Design review of the part built by this model. Coordinates are the model's own, in mm. Give positions to 0.01 mm unless a question says otherwise; leave off trailing zeros. Loops run counter-clockwise (first coordinate to the right, second up) from the corner with the lowest first, then second, coordinate; pieces in that order, holes last. Notation, with made-up numbers: (2.5, 32.25) -> (12.5, 32.25) arc R17 ccw to (12.5, 40.25) -> close; hole circle Ø3 at (32.5, 49). An arc over 180 degrees is marked (long way). Use a Markdown table: item, result. Add a question column.
1. Add section D-D (z = 2). State the section outline as (x, y) points.
2. For pin 1 Ø5 at (y, z) = (10, 6.5) entering from +X; pin 2 Ø4 at (y, z) = (6.5, -2) entering from +X, all flat-tipped, find the tip position at first contact; note any pin that passes through.
3. To check wall thickness, follow line 1 (Y direction, x = 55, z = -1.25); line 2 (Y direction, x = 55.5, z = 3); line 3 (X direction, y = 14.5, z = -4.5). State the ranges of each line that lie inside material, in increasing order.
4. Add section C-C (z = -1). State the section outline as (x, y) points.
5. Add section A-A (x = 55.3). State the section outline as (y, z) points, and give its area (3 significant figures).
6. Add section B-B (y = 11). State the section outline as (x, z) points, and give its area (3 significant figures).
```python
from build123d import *

# Parameters (mm, degrees)
BOSS_EXTRUDE1_DEPTH = 15
CUT_EXTRUDE1_DEPTH  = 40


with BuildPart() as part:
    # Sketch2 → Boss-Extrude1 (new body)
    with BuildSketch(Plane(origin=(0, 0, 0), x_dir=(1, 0, 0), z_dir=(0, 1, 0))):
        with BuildLine():
            Line((54.845806585, -8.617162068), (54.845806585, -10))
            ThreePointArc((54.845806585, -10), (55.523491502, -5.020397537), (55.75, 0))
            Line((55.75, 0), (55.518627344, 0))
            ThreePointArc((55.518627344, 0), (55.350166573, -4.321694398), (54.845806585, -8.617162068))
        make_face()
        with BuildLine():
            ThreePointArc((55.75, 0), (55.523491502, 5.020397537), (54.845806585, 10))
            Line((54.845806585, 10), (54.845806585, 8.617162068))
            ThreePointArc((54.845806585, 8.617162068), (55.350166573, 4.321694398), (55.518627344, 0))
            Line((55.518627344, 0), (55.75, 0))
        make_face()
        with BuildLine():
            Line((54.845806585, 8.617162068), (54.845806585, 0))
            Line((54.845806585, 0), (55.518627344, 0))
            ThreePointArc((55.518627344, 0), (55.350166573, 4.321694398), (54.845806585, 8.617162068))
        make_face()
        with BuildLine():
            Line((55.518627344, 0), (54.845806585, 0))
            Line((54.845806585, 0), (54.845806585, -8.617162068))
            ThreePointArc((54.845806585, -8.617162068), (55.350166573, -4.321694398), (55.518627344, 0))
        make_face()
    extrude(amount=BOSS_EXTRUDE1_DEPTH)

    # Sketch3 → Cut-Extrude1 (cut)
    with BuildSketch(Plane.ZY.offset(-43.464559905)):
        with BuildLine():
            ThreePointArc((0, 11.5), (-4, 7.5), (0, 3.5))
            Line((0, 3.5), (0, 7.5))
            Line((0, 7.5), (0, 11.5))
        make_face()
        with BuildLine():
            Line((0, 7.5), (0, 3.5))
            ThreePointArc((0, 3.5), (2.828427125, 4.671572875), (4, 7.5))
            Line((4, 7.5), (0, 7.5))
        make_face()
        with BuildLine():
            Line((0, 11.5), (0, 7.5))
            Line((0, 7.5), (4, 7.5))
            ThreePointArc((4, 7.5), (2.828427125, 10.328427125), (0, 11.5))
        make_face()
    extrude(amount=-CUT_EXTRUDE1_DEPTH, mode=Mode.SUBTRACT)


solid = part.part
```
Taken from the geometry:
| question | item | result |
|---|---|---|
| 1 | outline | (54.85, 0) -> (55.71, 0) -> (55.71, 4.04) -> (54.85, 4.04) -> close; (54.85, 10.96) -> (55.71, 10.96) -> (55.71, 15) -> (54.85, 15) -> close |
| 2 | pin 1 | stops at x = 55.61 |
| 2 | pin 2 | stops at x = 55.68 |
| 3 | line 1 | y = 0 to 3.7, 11.3 to 15 |
| 3 | line 2 | y = 0 to 4.85, 10.15 to 15 |
| 3 | line 3 | x = 54.85 to 55.57 |
| 4 | outline | (54.85, 0) -> (55.74, 0) -> (55.74, 3.63) -> (54.85, 3.63) -> close; (54.85, 11.37) -> (55.74, 11.37) -> (55.74, 15) -> (54.85, 15) -> close |
| 5 | outline | (0, -7.07) -> (15, -7.07) -> (15, 7.07) -> (0, 7.07) -> close; hole circle Ø8 at (7.5, 0) |
| 5 | area | 162 mm^2 |
| 6 | outline | (54.85, -10) arc R55.75 ccw to (55.72, -1.94) -> (54.85, -1.94) -> close; (54.85, 1.94) -> (55.72, 1.94) arc R55.75 ccw to (54.85, 10) -> close |
| 6 | area | 8.62 mm^2 |
